Can you work these out from the model? Positions are in its coordinate system, mm. Face numbers are marked on the shaded views. A direction names the side the tool comes from. Round coordinates to 2 decimals unless told otherwise and drop trailing zeros. Loops run counter-clockwise (first coordinate to the right, second up) from the corner with the lowest first, then second, coordinate; pieces in that order, holes last.
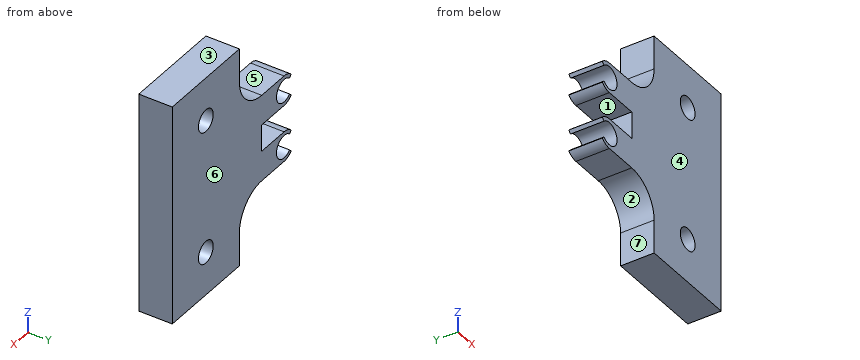
Autodesk Inventor part; units mm, degrees
ref_plane "YZ Plane" through (0, 0, 0) normal (1, 0, 0) x (0, 1, 0)
ref_plane "XZ Plane" through (0, 0, 0) normal (0, 1, 0) x (-1, 0, 0)
ref_plane "XY Plane" through (0, 0, 0) normal (0, 0, 1) x (1, 0, 0)
sketch "Sketch1" plane through (0, 0, 0) normal (0, 1, 0) x (-1, 0, 0)
  arc A0 (1.2021, 1.2021) -> (1.2021, -1.2021) centre (0, 0) ccw
  arc A1 (1.591, 1.591) -> (1.591, -1.591) centre (0, 0) ccw
  line L0 (0, 2.25) -> (0, 1.7)
  line L1 (0, -1.7) -> (0, -2.25)
  line L2 (0, 0) -> (1.2021, -1.2021)
  line L3 (0, 0) -> (1.7, 0) construction
  line L4 (0, 0) -> (1.2021, 1.2021)
  line L5 (1.2021, -1.2021) -> (1.591, -1.591)
  line L6 (1.2021, 1.2021) -> (1.591, 1.591)
  line L7 (0, 2.25) -> (-5, 2.25)
  line L8 (-5, 2.25) -> (-5, -2.25)
  line L9 (-5, -2.25) -> (0, -2.25)
  line L10 (0, 0) -> (0, -8.5)
  arc A2 (1.2021, -7.2979) -> (1.2021, -9.7021) centre (0, -8.5) ccw
  arc A3 (1.591, -6.909) -> (1.591, -10.091) centre (0, -8.5) ccw
  line L11 (0, -8.5) -> (1.2021, -9.7021)
  line L12 (0, -8.5) -> (1.7, -8.5) construction
  line L13 (0, -8.5) -> (1.2021, -7.2979)
  line L14 (0, -8.5) -> (1.7, -8.5) construction
  line L15 (1.2021, -9.7021) -> (1.591, -10.091)
  line L16 (1.2021, -7.2979) -> (1.591, -6.909)
  line L17 (0, -6.25) -> (-5, -6.25)
  line L18 (0, -10.75) -> (-5, -10.75)
  line L19 (-5, -10.75) -> (-5, -6.25)
  line L20 (-5, -2.25) -> (-5, -6.25)
  line L21 (0, -2.25) -> (-5, -2.25)
  line L22 (-5, -2.25) -> (-5, -6.25)
  line L23 (-5, -6.25) -> (0, -6.25)
  line L24 (0, -6.25) -> (0, -2.25)
  arc A4 (-10, 7.25) -> (-5, 2.25) centre (-5, 7.25) ccw
  arc A5 (-5, -10.75) -> (-10, -15.75) centre (-5, -15.75) ccw
  line L25 (-10, -15.75) -> (-10, -20.75)
  line L26 (-10, 7.25) -> (-10, 12.25)
  line L27 (-10, -20.75) -> (-25, -20.75)
  line L28 (-10, 12.25) -> (-25, 12.25)
  line L29 (-25, 12.25) -> (-25, -20.75)
  line L30 (-5, -4.25) -> (-17.5, -4.25)
  line L31 (-17.5, -4.25) -> (-17.5, -14.25)
  line L32 (-17.5, -4.25) -> (-17.5, 5.75)
  circle A6 centre (-17.5, 5.75) radius 1.65
  circle A7 centre (-17.5, -14.25) radius 1.65
  dimension "d0" = 3.4
  dimension "d1" = 4.5
  dimension "d2" = 45
  dimension "d5" = 5
  dimension "d6" = 8.5
  dimension "d7" = 3.4
  dimension "d8" = 4.5
  dimension "d9" = 45
  dimension "d10" = 45
  dimension "d15" = 5
  dimension "d16" = 5
  dimension "d17" = 15
  dimension "d18" = 15
  dimension "d19" = 10
  dimension "d20" = 10
  dimension "d21" = 3.3
  dimension "d22" = 3.3
extrude "Extrusion3" add sketch "Sketch1" along normal blind 5 contours A0 L0 A1 L6 | A0 L1 A1 L0 | A0 L5 A1 L1 | A1 L9 L8 L7 | L8 L20 L19 A5 L25 L27 L29 L28 L26 A4 | A3 L16 A2 L10 | L10 A2 L15 A3 | A3 L18 L19 L17
properties part number "headphonesclip"
(1) For pin 1 (1 mm diameter, centred on x = 19.5, z = -1, fed in from -Y); pin 2 (2 mm diameter, centred on x = 5, y = 1.5, fed in from -Z); pin 3 (2.5 mm diameter, centred on y = 2, z = -18, fed in from -X); pin 4 (1.5 mm diameter, centred on x = 2, y = 3, fed in from +Z), each with a flat end and sliding along its axis, tell me the tip position at first contact or that it passes through.
(2) Suppose I cut it at C-C (y = 0.4). Write out the boundary of the cut face in (x, z), then the cut area to 3 significant figures.
(3) Suppose I cut it at A-A (x = 17.5). Write out the boundary of the cut face in (y, z).
(4) Suppose I cut it at D-D (z = -14.25). Write out the boundary of the cut face in (x, y).
(5) If I drill on line 1 (Z direction, x = 17.5, y = 1.85); line 2 (Z direction, x = 0, y = 2.95); line 3 (Z direction, x = 4.5, y = 1.05), over which ranges is the centre line in solid material (lowest first)?
(6) We'd pull the mould along Z, two halves only. Please class the marked faces 1, 2, 3 and 4: released by +Z, released by -Z, zero draft, split by the parting line, or undercut.
(7) Suppose I cut it at B-B (x = 3.25). Write out the boundary of the cut face in (y, z), then the cut area to 3 significant figures.
(8) Which directions (+Z, -Z, +X, -X, +Y, -Y) give clear straight access to the entire face, cutting with the end or side of a thin tool? Please do the marked faces 5, 6 and 7.
Check result:
1. pin 1: stops at y = 0
1. pin 2: stops at z = -10.85
1. pin 3: stops at x = 10
1. pin 4: stops at z = 2.25
2. outline: (-1.59, -10.09) arc R2.25 ccw to (0, -10.75) - (5, -10.75) arc R5 cw to (10, -15.75) - (10, -20.75) - (25, -20.75) - (25, 12.25) - (10, 12.25) - (10, 7.25) arc R5 cw to (5, 2.25) - (0, 2.25) arc R2.25 ccw to (-1.59, 1.59) - (-1.2, 1.2) arc R1.7 cw (long way) to (-1.2, -1.2) - (-1.59, -1.59) arc R2.25 ccw to (0, -2.25) - (5, -2.25) - (5, -6.25) - (0, -6.25) arc R2.25 ccw to (-1.59, -6.91) - (-1.2, -7.3) arc R1.7 cw (long way) to (-1.2, -9.7) - close; hole circle Ø3.3 at (17.5, -14.25); hole circle Ø3.3 at (17.5, 5.75)
2. area: 593 mm2
3. outline: (0, -20.75) - (5, -20.75) - (5, -15.9) - (0, -15.9) - close; (0, -12.6) - (5, -12.6) - (5, 4.1) - (0, 4.1) - close; (0, 7.4) - (5, 7.4) - (5, 12.25) - (0, 12.25) - close
4. outline: (9.77, 0) - (15.85, 0) - (15.85, 5) - (9.77, 5) - close; (19.15, 0) - (25, 0) - (25, 5) - (19.15, 5) - close
5. line 1: z = -20.75 to -15.9, -12.6 to 4.1, 7.4 to 12.25
5. line 2: z = -10.75 to -10.2, -6.8 to -6.25, -2.25 to -1.7, 1.7 to 2.25
5. line 3: z = -10.75 to -6.25, -2.25 to 2.25
6. face 1: undercut
6. face 2: released by -Z
6. face 3: released by +Z
6. face 4: zero draft
7. outline: (0, -10.75) - (5, -10.75) - (5, -6.25) - (0, -6.25) - close; (0, -2.25) - (5, -2.25) - (5, 2.25) - (0, 2.25) - close
7. area: 45.0 mm2
8. face 5: +Z, -X, +Y, -Y
8. face 6: +Z, -Z, +X, -X, +Y
8. face 7: -Z, -X, +Y, -Y
